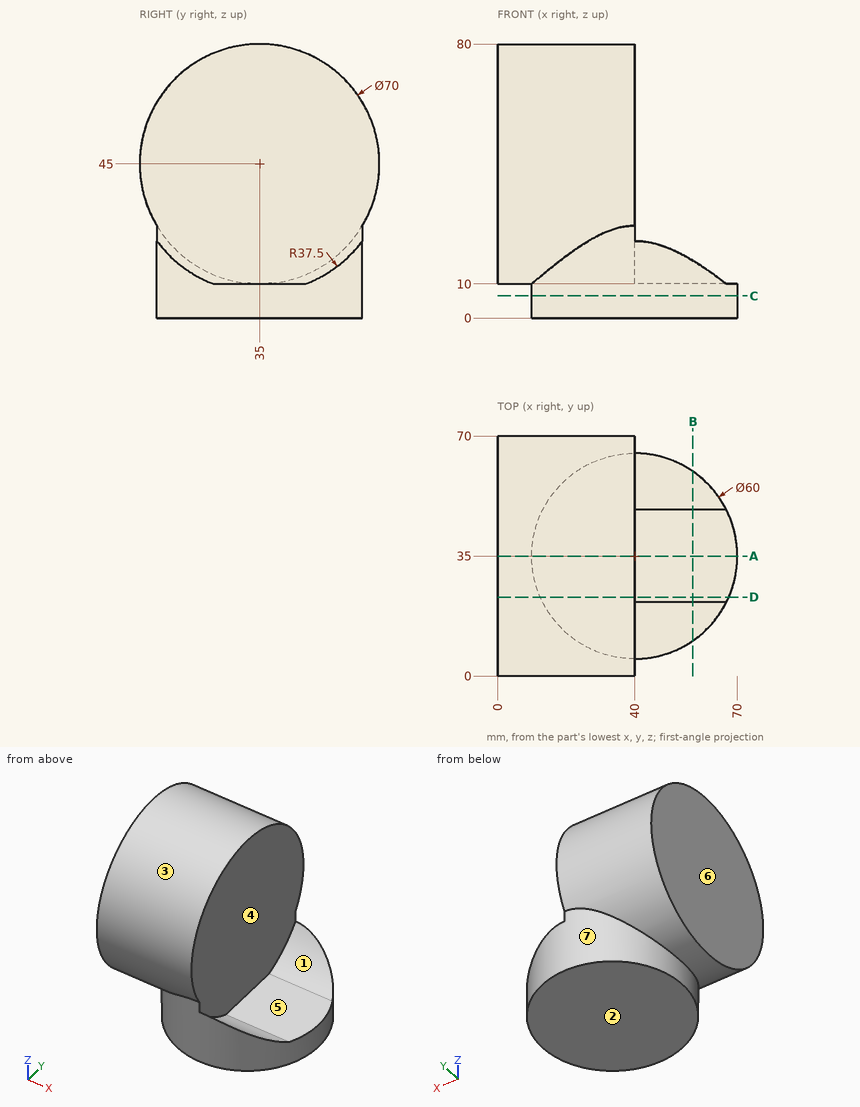
Print and shaded views of the part. All mm, measured from the part's lowest x, y and z. A direction names the side the tool comes from. Coordinates: 2 decimals unless noted, no trailing zeros. Order: outer loops, then holes, each group sorted by start corner. A loop starts at its lowest first (then second) coordinate and runs counter-clockwise, first axis right, second up.
(1) Slice it at B-B, the plane x = 57. Write the cut outline in (y, z).
Check sheet entries:
outline: (10.28, 0) - (59.72, 0) - (59.72, 16.8) arc R37.5 cw to (48.46, 10) - (21.54, 10) arc R37.5 cw to (10.28, 16.8) - close
(2) Tool access for the marked faces 5, 6 and 7: list every direction of +Z, -Z, +X, -X, +Y, -Y with a clear straight run to the whole face (end or side of a thin tool).
Check sheet entries:
face 5: +Z, +X
face 6: +Z, -Z, -X, +Y, -Y
face 7: -Z
(3) Slice it at C-C, the plane z = 6.5. Write the cut outline in (x, y), and give its area (3 significant figures).
Check sheet entries:
outline: circle Ø60 at (40, 35)
area: 2,830 mm2
(4) Slice it at D-D, the plane y = 23. Write the cut outline in (x, z).
Check sheet entries:
outline: (0, 12.12) - (12.5, 12.12) - (12.5, 0) - (67.5, 0) - (67.5, 10) - (40, 10) - (40, 77.88) - (0, 77.88) - close
(5) Slice it at A-A, the plane y = 35. Write the cut outline in (x, z), and give its area (3 significant figures).
Check sheet entries:
outline: (0, 10) - (10, 10) - (10, 0) - (70, 0) - (70, 10) - (40, 10) - (40, 80) - (0, 80) - close
area: 3,400 mm2
(6) Pin check, flat tips, straight feed: pin 1 Ø3 at (x, y) = (32, 33.5) entering from +Z; pin 2 Ø8 at (x, z) = (35.5, 70) entering from -Y; pin 3 Ø5 at (x, z) = (41.5, 55.5) entering from -Y. Stop position of each tip, or through.
Check sheet entries:
pin 1: stops at z = 80
pin 2: stops at y = 7
pin 3: stops at y = 1.05
(7) Probe L1, parallel to X at y = 38, z = 48; L2, parallel to Z at x = 48.5, y = 47.5; L3, parallel to X at y = 13, z = 6. List the from-to ranges inside material, lowest first.
Check sheet entries:
L1: x = 0 to 40
L2: z = 0 to 10
L3: x = 19.6 to 60.4
(8) Pull direction Y, two halves, no side cores. Call the marked faces 1, 2, 3 and 4: pulls with the +Y half, pulls with the -Y half, needs draft (parallel to the pull), parting line crosses it, or undercut.
Check sheet entries:
face 1: undercut
face 2: needs draft
face 3: parting line crosses it
face 4: undercut
